Part model, mm, in its own coordinate system. Face numbers are marked on the shaded views. A direction names the side the tool comes from. Coordinates: 2 decimals unless noted, no trailing zeros. Loops run counter-clockwise (first coordinate to the right, second up) from the corner with the lowest first, then second, coordinate; pieces in that order, holes last. Notation, with made-up numbers: M 86,81.25 L 93,81.25 A26 cw 93,103.25 Z; hole C 71,-28 d10. An arc over 180 degrees is marked long. Use CSV: the item, a comma, the result in double quotes. Start each with the question number.
Autodesk Fusion 360 part; units mm, degrees
sketch "Sketch1" plane through (0, 0, 0) normal (0, 0, 1) x (1, 0, 0)
  circle A0 centre (0, 0) radius 31
  dimension "d1" = 62
extrude "Extrude1" add sketch "Sketch1" along normal blind 55
sketch "Sketch2" plane through (0, 0, 55) normal (0, 0, 1) x (-1, 0, 0)
  circle A0 centre (0, 0) radius 31
  circle A1 centre (0, 0) radius 16.25
  dimension "d4" = 32.5
extrude "Extrude2" cut sketch "Sketch2" against normal blind 50 contours A1
sketch "Sketch3" plane through (0, 0, 55) normal (0, 0, 1) x (-1, 0, 0)
  circle A0 centre (0, 0) radius 16.25
  circle A1 centre (0, 0) radius 31
  line L0 (10, -25) -> (-10, -25)
  line L1 (-10, -25) -> (-10, 25)
  line L2 (-10, 25) -> (10, 25)
  line L3 (10, 25) -> (10, -25)
  line L4 (10, -25) -> (-10, 25) construction
  line L5 (-10, -25) -> (10, 25) construction
  dimension "d7" = 20
  dimension "d8" = 50
extrude "Extrude3" cut sketch "Sketch3" against normal blind 50 contours A0 L1 L2 L3 | A0 L0 L1 L3
sketch "Sketch4" plane through (0, -25, 0) normal (0, 1, 0) x (-1, 0, 0)
  line L0 (10, 55) -> (-10, 55)
  line L1 (-10, 55) -> (-10, 5)
  line L2 (-10, 5) -> (10, 5)
  line L3 (10, 5) -> (10, 55)
  line L4 (5, 12.5) -> (-5, 12.5)
  line L5 (-5, 12.5) -> (-5, 7.5)
  line L6 (-5, 7.5) -> (5, 7.5)
  line L7 (5, 7.5) -> (5, 12.5)
  line L8 (5, 12.5) -> (-5, 7.5) construction
  line L9 (-5, 12.5) -> (5, 7.5) construction
  point P0 (0, 10)
  dimension "d11" = 10
  dimension "d12" = 5
extrude "Extrude4" cut sketch "Sketch4" against normal blind 8 contours L4 L5 L6 L7
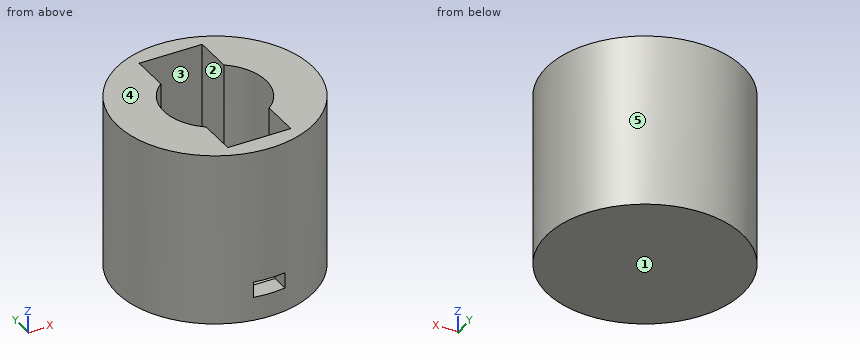
1. Slice it at A-A, the plane x = 0. List the corners of the cut face in (y, z), and give its area (3 significant figures).
2. Tool access for the marked faces 1 and 2: list every direction of +Z, -Z, +X, -X, +Y, -Y with a clear straight run to the whole face (end or side of a thin tool).
3. Slice it at D-D, the plane y = -26.5. List the corners of the cut face in (x, z).
4. Pin check, flat tips, straight feed: pin 1 (13.5 mm diameter, centred on y = 18, z = 36, fed in from -X); pin 2 (3.5 mm diameter, centred on y = -17, z = 35, fed in from +X); pin 3 (1 mm diameter, centred on y = 12, z = 29, fed in from -X). Stop position of each tip, or through.
5. Wall check: probe 1 along Y at (x, z) = (-1, 40.5); probe 2 along Z at (x, y) = (12.5, -3); probe 3 along X at (y, z) = (3, 19). Give the ranges that are in metal, low to high.
6. Two-plate mould, pull along X, no slides. Class the marked faces 3, 4 and 5: pulls with the +X half, pulls with the -X half, needs draft (parallel to the pull), parting line crosses it, or undercut.
7. Slice it at B-B, the plane z = 34. List the corners of the cut face in (x, y).
8. Slice it at C-C, the plane y = 0. List the corners of the cut face in (x, z).
Found:
1,outline,"M -31,0 L 31,0 L 31,55 L 25,55 L 25,5 L -25,5 L -25,7.5 L -31,7.5 Z; M -31,12.5 L -25,12.5 L -25,55 L -31,55 Z"
1,area,"880 mm^2"
2,face 1,"-Z, +X, -X, +Y, -Y"
2,face 2,"+Z"
3,outline,"M -16.09,0 L 16.09,0 L 16.09,55 L -16.09,55 Z; hole M -5,7.5 L 5,7.5 L 5,12.5 L -5,12.5 Z"
4,pin 1,"x = -28.89"
4,pin 2,"x = 26.99"
4,pin 3,"x = -28.79"
5,probe 1,"-30.98 to -25, 25 to 30.98"
5,probe 2,"0 to 5"
5,probe 3,"-30.85 to -15.97, 15.97 to 30.85"
6,face 3,"undercut"
6,face 4,"needs draft"
6,face 5,"parting line crosses it"
7,outline,"C 0,0 d62; hole M -10,-25 L 10,-25 L 10,-12.81 A16.25 ccw 10,12.81 L 10,25 L -10,25 L -10,12.81 A16.25 ccw -10,-12.81 Z"
8,outline,"M -31,0 L 31,0 L 31,55 L 16.25,55 L 16.25,5 L -16.25,5 L -16.25,55 L -31,55 Z"
